Here's how the part is built. I have some questions about the finished solid (model axes, mm). Face numbers are marked on the shaded views. A direction names the side the tool comes from. Round coordinates to 2 decimals unless told otherwise and drop trailing zeros. Loops run counter-clockwise (first coordinate to the right, second up) from the corner with the lowest first, then second, coordinate; pieces in that order, holes last. Notation, with made-up numbers: M -3,-34 L 14,-34 A24 cw 14,-18 Z; hole C -8.5,-26 d8. An arc over 180 degrees is marked long. Put each result on its own line as item: value. Start each with the question number.
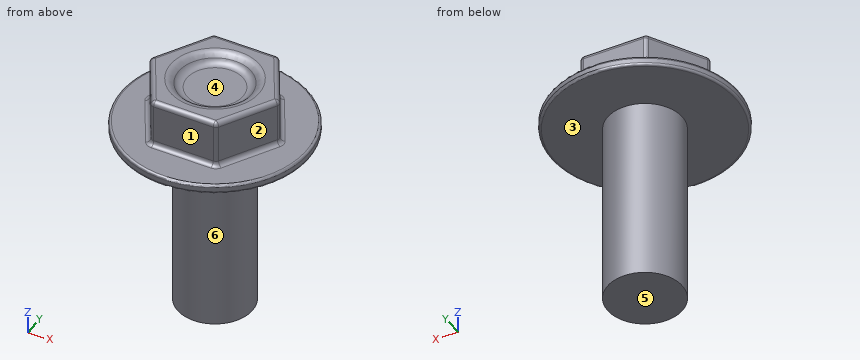
```python
from build123d import *

# Parameters (mm, degrees)
SKETCH1_R           = 8
BOSS_EXTRUDE1_DEPTH = 40
SKETCH1_3_R         = 20
BOSS_EXTRUDE2_DEPTH = 2
BOSS_EXTRUDE3_DEPTH = 10
CUT_EXTRUDE1_START  = 10
SKETCH2_3_R         = 8
CUT_EXTRUDE1_DEPTH  = 2
FILLET1_R           = 0.5
FILLET2_R           = 1
FILLET3_R           = 2
FILLET4_R           = 2


with BuildPart() as part:
    # Sketch1 → Boss-Extrude1 (new body)
    with BuildSketch(Plane(origin=(0, 0, 0), x_dir=(0, 1, 0), z_dir=(0, 0, 1))):
        with Locations(Location((0, 0, 0), (0, 0, 270))):
            Circle(SKETCH1_R)
    extrude(amount=-BOSS_EXTRUDE1_DEPTH)

    # Sketch1<3> → Boss-Extrude2 (add)
    with BuildSketch(Plane(origin=(0, 0, 0), x_dir=(0, 1, 0), z_dir=(0, 0, 1))):
        with Locations(Location((0, 0, 0), (0, 0, 270))):
            Circle(SKETCH1_3_R)
    extrude(amount=BOSS_EXTRUDE2_DEPTH)

    # Sketch2 → Boss-Extrude3 (add)
    with BuildSketch(Plane.XY.offset(2)):
        Polygon((-14, 0), (-7, -12.124355653), (7, -12.124355653), (14, 0), (7, 12.124355653), (-7, 12.124355653), align=None)
    extrude(amount=BOSS_EXTRUDE3_DEPTH)

    # Sketch2<3> → Cut-Extrude1 (cut)
    with BuildSketch(Plane.XY.offset(2).offset(CUT_EXTRUDE1_START)):
        Circle(SKETCH2_3_R)
    extrude(amount=-CUT_EXTRUDE1_DEPTH, mode=Mode.SUBTRACT)

    # Fillet1
    fillet1_edges = [part.edges().sort_by_distance(p)[0] for p in [
        (-20, 0, 0),
        (-20, 0, 2),
    ]]
    fillet(fillet1_edges, radius=FILLET1_R)

    # Fillet2
    fillet2_edges = [part.edges().sort_by_distance(p)[0] for p in [
        (0, -12.124355653, 2),
        (-7, -12.124355653, 7),
        (10.5, -6.062177826, 2),
        (7, -12.124355653, 7),
        (10.5, 6.062177826, 2),
        (14, 0, 7),
        (0, 12.124355653, 2),
        (7, 12.124355653, 7),
        (-10.5, 6.062177826, 2),
        (-7, 12.124355653, 7),
        (-10.5, -6.062177826, 2),
        (-14, 0, 7),
        (0, -12.124355653, 12),
        (10.5, -6.062177826, 12),
        (10.5, 6.062177826, 12),
        (0, 12.124355653, 12),
        (-10.5, 6.062177826, 12),
        (-10.5, -6.062177826, 12),
    ]]
    fillet(fillet2_edges, radius=FILLET2_R)

    # Fillet3
    fillet3_edges = [part.edges().sort_by_distance(p)[0] for p in [
        (-8, 0, 10),
    ]]
    fillet(fillet3_edges, radius=FILLET3_R - 0.0001)  # a hair under: the kernel refuses the full size

    # Fillet4
    fillet4_edges = [part.edges().sort_by_distance(p)[0] for p in [
        (-8, 0, 12),
    ]]
    fillet(fillet4_edges, radius=FILLET4_R)


solid = part.part
```
1) If I drill on probe 1 along Z at (x, y) = (-5, -10.5); probe 2 along Z at (x, y) = (10, 13); probe 3 along X at (y, z) = (-5, 7.5), over which ranges is the centre line in solid material (lowest first)? Write a range as from..to.
2) On a 3-axis mill with a long thin cutter (end or side, diameter ignored), from which of +Z, -Z, +X, -X, +Y, -Y can I reach the whole of each face in a straight line? I mean the marked faces 1, 2 and 3. Say none if no direction works.
3) I'm going to push flat-ended pins straight in: P1, Ø6, axis at x = -6, z = -0.5, coming from the +Y side; P2, Ø4, axis at x = 10.5, z = 5, coming from the +Y side; P3, Ø6.5, axis at x = -2.5, z = 6, coming from the -Y side; P4, Ø1, axis at y = -11.5, z = -2, coming from the -X side. Where does each tip first touch, or does it pass through?
4) Suppose I cut it at A-A (z = 4). Write out the boundary of the cut face in (x, y), plus the area to 3 significant figures.
5) If we mould it in two halves opening along Y, with no side actions, what happens to the marked faces 4, 5 and 6? For each: pulls with the +Y half, pulls with the -Y half, needs draft (parallel to the pull), parting line crosses it, or undercut.
6) Suppose I cut it at B-B (z = -21). Write out the boundary of the cut face in (x, y), plus the area to 3 significant figures.
Results are:
1. probe 1: 0..12
1. probe 2: 0..2
1. probe 3: -11.11..11.11
2. face 1: +Z, +X, -X, -Y
2. face 2: +Z, +X, -Y
2. face 3: -Z
3. P1: y = 19.75
3. P2: y = 9.53
3. P3: y = -12.16
3. P4: through
4. outline: M -13.71,-0.5 L -7.29,-11.62 A1 ccw -6.42,-12.12 L 6.42,-12.12 A1 ccw 7.29,-11.62 L 13.71,-0.5 A1 ccw 13.71,0.5 L 7.29,11.62 A1 ccw 6.42,12.12 L -6.42,12.12 A1 ccw -7.29,11.62 L -13.71,0.5 A1 ccw Z
4. area: 509 mm²
5. face 4: undercut
5. face 5: needs draft
5. face 6: parting line crosses it
6. outline: C 0,0 d16
6. area: 201 mm²
